Geometry: see drawing. Coordinates: mm, zero at the bounding-box minimum. A direction names the side the tool comes from. Coordinates: 2 decimals unless noted, no trailing zeros. Write each loop counter-clockwise with the first axis right and the second up, starting at its lowest first coordinate (ties: lowest second). Pieces come first, ordered by that corner, then holes. Notation, with made-up numbers: M -15.75,-40 L 8.25,-40 A34 cw 8.25,-1 Z; hole C 59,40 d4. An arc over 180 degrees is marked long. One line per item, written item: value. Start each with the question number.
Item 1: Mould query, pull axis X, two halves, no side actions, for the marked faces 4, 5 and 6. Classes: released by +X, released by -X, zero draft, split by the parting line, or undercut.
Item 2: Cut plane B-B, the plane x = 21. State how many separate pieces and enclosed holes the cut face has, then the cut area to 3 significant figures.
Item 3: Pin query (flat end, axial travel): P1, Ø1, axis at y = 2.5, z = 25.5, coming from the -X side (1 decimal); P2, Ø2, axis at x = 35.5, y = 3, coming from the -Z side; P3, Ø1.9, axis at x = 17, y = 3, coming from the -Z side. Return the tip coordinate at first contact, or that it passes through.
Item 4: Ray query, L1, parallel to X at y = 5, z = 21 (1 decimal); L2, parallel to Z at x = 13.5, y = 4.25 (1 decimal); L3, parallel to Z at x = 14, y = 5.25 (1 decimal). Return the intervals inside material, ascending. Write a range as from..to.
Item 5: Set-up query: the marked faces 1, 2 and 3. Return all of +Z, -Z, +X, -X, +Y, -Y with unobstructed straight access to the full face (end or side cutting, diameter ignored); none if empty.
Item 6: Cut plane A-A, the plane z = 29. Output: boundary loops of the cut face in (x, y).
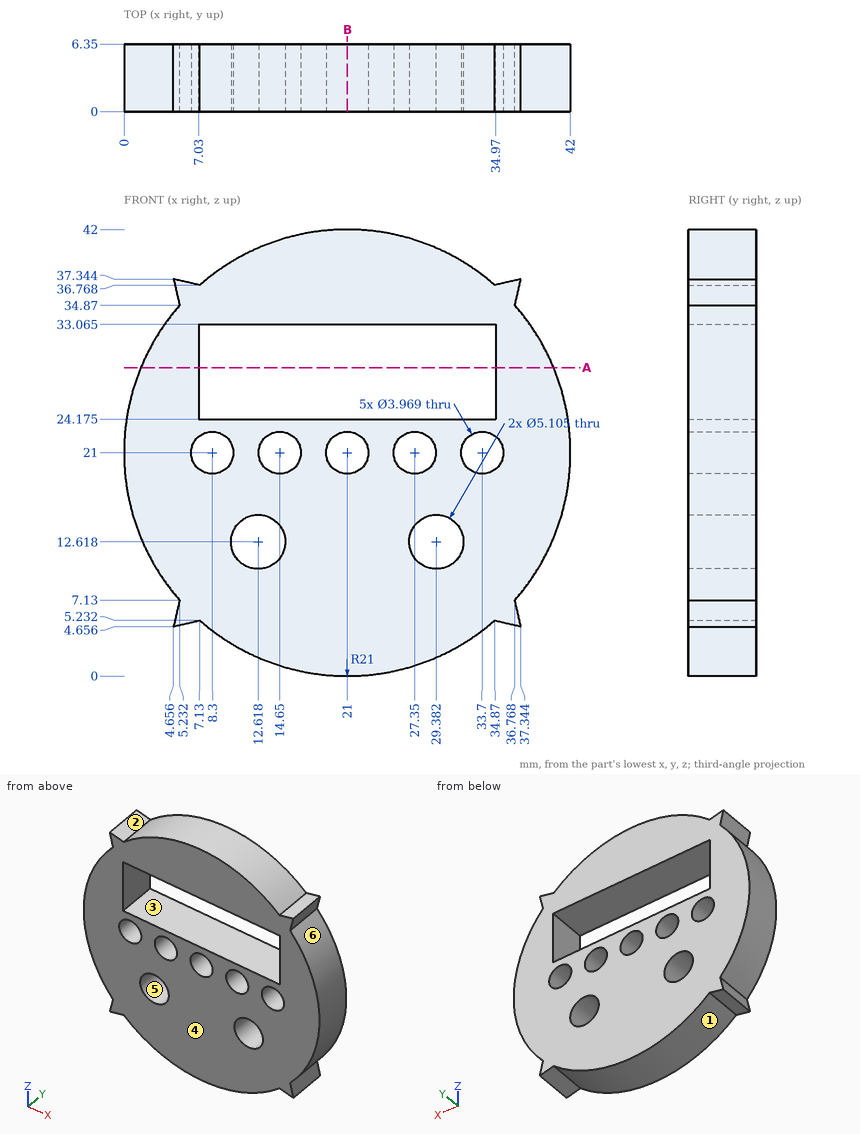
From the geometry:
1. face 4: zero draft
1. face 5: undercut
1. face 6: released by +X
2. separate pieces: 3
2. enclosed holes: 0
2. area: 185 mm²
3. P1: stops at x = 0.4
3. P2: stops at z = 4.85
3. P3: stops at z = 0.22
4. L1: x = 0..6.3, 10.3..12.7, 16.6..19, 23..25.4, 29.3..31.7, 35.7..42
4. L2: z = 1.4..10.2, 15..19.4, 22.6..24.2, 33.1..40.6
4. L3: z = 1.2..10.5, 14.8..19.1, 22.9..24.2, 33.1..40.8
5. face 1: -Z, +Y, -Y
5. face 2: +Z, +Y, -Y
5. face 3: +Y, -Y
6. outline: M 1.58,0 L 7.03,0 L 7.03,6.35 L 1.58,6.35 Z; M 34.97,0 L 40.42,0 L 40.42,6.35 L 34.97,6.35 Z
